Design review of the part built by this model. Coordinates are the model's own, in mm. A direction names the side the tool comes from. Coordinates: 2 decimals unless noted, no trailing zeros. Write each loop counter-clockwise with the first axis right and the second up, starting at its lowest first coordinate (ties: lowest second). Pieces come first, ordered by that corner, then holes.
Q1. Machinability: for faces 1 (the face through (7, 0, 10.788)), 2 (the face through (5.715, 0, 19)), 3 (the face through (0, 6.35, 0)), 4 (the face through (5.715, 0, 0)), 5 (the face through (-5.715, 0, 19)), which of the approach directions +Z, -Z, +X, -X, +Y, -Y give a long, thin tool a straight path to every point of the face, cutting with its end or side? Answer none if there is none.
Q2. Add section B-B, the plane x = -7. Give the boundary of the cut face in (y, z), plus the area to 3 significant figures.
Q3. To check wall thickness, follow probe 1 along Z at (x, y) = (-4.25, -5.75) (3 decimals); probe 2 along Z at (x, y) = (-5.75, -9); probe 3 along X at (y, z) = (-5.25, -1) (3 decimals). State the ranges of each line that lie inside material, in increasing order.
Q4. Clearance check with flat-ended pins moving along their axes: pin 1 Ø7 at (y, z) = (-1, -1.5) entering from +X (3 decimals); pin 2 Ø4 at (x, z) = (2, 2) entering from -Y; pin 3 Ø1 at (x, z) = (-3.5, 14) entering from -Y. State where each tip first meets the part, or that it passes through.
Q5. Add section A-A, the plane z = -2.25. Give the boundary of the cut face in (x, y) (3 decimals).
Solid Edge part; units mm, degrees
sketch "Sketch1" plane through (0, 0, 0) normal (1, 0, 0) x (0, 1, 0)
  line L0 (-6.35, -4.445) -> (-6.35, 4.445)
  line L1 (-6.35, 4.445) -> (6.35, 4.445)
  line L2 (6.35, 4.445) -> (6.35, -4.445)
  line L3 (6.35, -4.445) -> (-6.35, -4.445)
extrude "Protrusion1" add sketch "Sketch1" along normal mid plane 11.43
sketch "Sketch2" plane through (0, 0, 11.938) normal (0, 0, 1) x (1, 0, 0)
  line L0 (6.35, -7.8613) -> (-6.35, -7.8613)
  line L1 (-6.35, -7.8613) -> (-6.35, 7.8613)
  line L2 (-6.35, 7.8613) -> (6.35, 7.8613)
  line L3 (6.35, 7.8613) -> (6.35, -7.8613)
sketch "Sketch3" plane through (0, 0, 4.445) normal (0, 0, 1) x (0, -1, 0)
  line L0 (6.35, 5.715) -> (-6.35, 5.715)
  line L1 (-6.35, 5.715) -> (-6.35, -5.715)
  line L2 (6.35, -5.715) -> (-6.35, -5.715)
  line L3 (6.35, 5.715) -> (6.35, -5.715)
loft "LoftedProtrusion1" add profiles "Sketch2", "Sketch3"
sketch "Sketch4" plane through (0, 0, 11.938) normal (0, 0, 1) x (-1, 0, 0)
  line L0 (-7.8994, 9.9187) -> (-7.8994, -9.9187)
  line L1 (-7.8994, -9.9187) -> (7.8994, -9.9187)
  line L2 (7.8994, -9.9187) -> (7.8994, 9.9187)
  line L3 (7.8994, 9.9187) -> (-7.8994, 9.9187)
extrude "ExtrudedProtrusion_2" add sketch "Sketch4" along normal mid plane 2.3
sketch "Sketch5" plane through (0, 0, 0) normal (1, 0, 0) x (0, 1, 0)
  line L0 (-1, 24.631) -> (-1.5, 13.7696)
  line L1 (-1.5, 13.7696) -> (-2.1816, 13.088)
  line L2 (-2.1816, 13.088) -> (2.1816, 13.088)
  line L3 (2.1816, 13.088) -> (1.5, 13.7696)
  line L4 (1.5, 13.7696) -> (1, 24.631)
  line L5 (-1, 24.631) -> (1, 24.631)
extrude "ExtrudedProtrusion_3" add sketch "Sketch5" along normal mid plane 11.43
Here are the results:
1. face 1: -Z
1. face 2: +Z, +X, +Y, -Y
1. face 3: -Z, +X, -X, +Y
1. face 4: -Z, +X, +Y, -Y
1. face 5: +Z, -X, +Y, -Y
2. outline: (-9.92, 10.79) - (9.92, 10.79) - (9.92, 13.09) - (-9.92, 13.09) - close
2. area: 45.6 mm2
3. probe 1: z = -4.445 to 13.088
3. probe 2: z = 10.79 to 13.09
3. probe 3: x = -5.715 to 5.715
4. pin 1: stops at x = 5.715
4. pin 2: stops at y = -6.35
4. pin 3: stops at y = -1.77
5. outline: (-5.715, -6.35) - (5.715, -6.35) - (5.715, 6.35) - (-5.715, 6.35) - close
